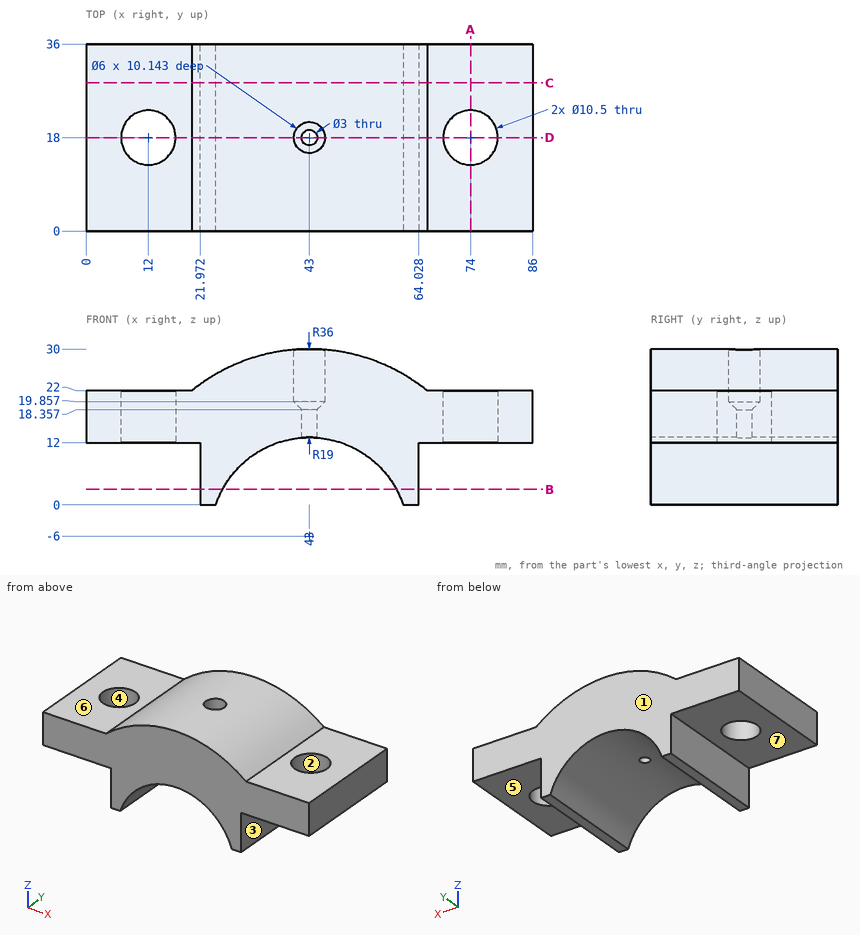
Part print with two shaded views. Sizes in mm from the minimum x, y, z corner. A direction names the side the tool comes from. Give positions to 0.01 mm unless a question says otherwise; leave off trailing zeros. Order: outer loops, then holes, each group sorted by start corner. A loop starts at its lowest first (then second) coordinate and runs counter-clockwise, first axis right, second up.
1) Pin check, flat tips, straight feed: pin 1 (1 mm diameter, centred on x = 47, y = 9.5, fed in from +Z); pin 2 (16.5 mm diameter, centred on x = 7, y = 18.5, fed in from +Z); pin 3 (8 mm diameter, centred on y = 16, z = 26.5, fed in from +X) (1 decimal). Stop position of each tip, or through.
2) Saw through at D-D, the plane y = 18. Count the separate pieces of the cut face and the enclosed holes in it.
3) Mould opens along Y. For the marked faces 1, 2, 3 and 4 say: +Y half, -Y half, draft (parallel to the pull), parting line (faces both ways), or undercut.
4) Wall check: probe 1 along Y at (x, z) = (43, 16.6); probe 2 along Y at (x, z) = (74, 15); probe 3 along Z at (x, y) = (5, 15). Give the ranges that are in metal, low to high.
5) 3-axis set-ups, long thin cutter, end or side, ignore diameter. For the marked faces 5, 6 and 7: which of +Z, -Z, +X, -X, +Y, -Y reach the whole face in a straight line?
6) Saw through at C-C, the plane y = 28.5. Write the cut outline in (x, z).
7) Saw through at B-B, the plane z = 3. Write the cut outline in (x, y), then the cut area to 3 significant figures.
8) Saw through at A-A, the plane x = 74. Write the cut outline in (y, z), then the cut area to 3 significant figures.
Computed:
1. pin 1: stops at z = 29.83
1. pin 2: stops at z = 22
1. pin 3: stops at x = 65
2. separate pieces: 4
2. enclosed holes: 0
3. face 1: +Y half
3. face 2: undercut
3. face 3: draft
3. face 4: undercut
4. probe 1: y = 0 to 16.5, 19.5 to 36
4. probe 2: y = 0 to 12.75, 23.25 to 36
4. probe 3: z = 12 to 22
5. face 5: -Z, +X, +Y, -Y
5. face 6: +Z, -X, +Y, -Y
5. face 7: -Z, -X, +Y, -Y
6. outline: (0, 12) - (21.97, 12) - (21.97, 0) - (24.97, 0) arc R19 cw to (61.03, 0) - (64.03, 0) - (64.03, 12) - (86, 12) - (86, 22) - (65.63, 22) arc R36 ccw to (20.37, 22) - (0, 22) - close
7. outline: (21.97, 0) - (26.27, 0) - (26.27, 36) - (21.97, 36) - close; (59.73, 0) - (64.03, 0) - (64.03, 36) - (59.73, 36) - close
7. area: 309 mm2
8. outline: (0, 12) - (12.75, 12) - (12.75, 22) - (0, 22) - close; (23.25, 12) - (36, 12) - (36, 22) - (23.25, 22) - close
8. area: 255 mm2
